Read the model definition and answer for the solid it produces. Units are mm, in the model's axes. Give positions to 0.01 mm unless a question says otherwise; leave off trailing zeros. Order: outer loops, then holes, each group sorted by start corner. A loop starts at its lowest first (then second) coordinate and runs counter-clockwise, first axis right, second up. Notation, with made-up numbers: (66.25, 74) -> (74.25, 74) arc R20 ccw to (74.25, 88) -> close; hole circle Ø2 at (42, -16). An arc over 180 degrees is marked (long way). Use one line per item in the form item = value.
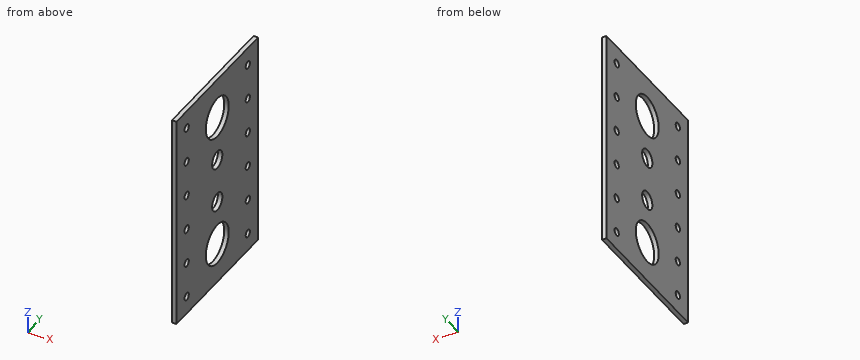
Autodesk Inventor part; units mm, degrees
ref_plane "YZ Plane" through (0, 0, 0) normal (1, 0, 0) x (0, 1, 0)
ref_plane "XZ Plane" through (0, 0, 0) normal (0, 1, 0) x (-1, 0, 0)
ref_plane "XY Plane" through (0, 0, 0) normal (0, 0, 1) x (1, 0, 0)
sketch "Sketch1" plane through (0, 0, 0) normal (1, 0, 0) x (0, 1, 0)
  line L0 (0, 0) -> (101.6, 0)
  line L1 (101.6, 0) -> (101.6, -152.4)
  line L2 (101.6, -152.4) -> (0, -152.4)
  line L3 (0, -152.4) -> (0, 0)
  circle A0 centre (50.8, -28.575) radius 14.2875
  circle A1 centre (50.8, -60.325) radius 6.35
  circle A2 centre (50.8, -92.075) radius 6.35
  circle A3 centre (50.8, -123.825) radius 14.2875
  line L4 (50.8, -28.575) -> (50.8, -123.825) construction
  circle A4 centre (88.9, -12.7) radius 2.65
  circle A5 centre (88.9, -38.1) radius 2.65
  circle A6 centre (88.9, -63.5) radius 2.65
  circle A7 centre (88.9, -88.9) radius 2.65
  circle A8 centre (88.9, -114.3) radius 2.65
  circle A9 centre (88.9, -139.7) radius 2.65
  circle A10 centre (12.7, -12.7) radius 2.65
  circle A11 centre (12.7, -38.1) radius 2.65
  circle A12 centre (12.7, -63.5) radius 2.65
  circle A13 centre (12.7, -88.9) radius 2.65
  circle A14 centre (12.7, -114.3) radius 2.65
  circle A15 centre (12.7, -139.7) radius 2.65
  point P0 (101.6, -76.2)
  point P1 (50.8, -76.2)
  point P2 (50.8, -152.4)
  dimension "d0" = 101.6
  dimension "d1" = 152.4
  dimension "d2" = 28.575
  dimension "d3" = 12.7
  dimension "d4" = 12.7
  dimension "d5" = 28.575
  dimension "d6" = 31.75
  dimension "d7" = 31.75
  dimension "d8" = 31.75
  dimension "d9" = 5.3
  dimension "d10" = 12.7
  dimension "d11" = 12.7
  dimension "d14" = 25.4
  dimension "d17" = 76.2
extrude "Extrusion1" add sketch "Sketch1" along normal blind 3.175
equation "\"d7\" = d6"
equation "\"d8\" = d7"
properties part number "CH-1-02-RearGearboxHousingMotorSide" material "Aluminum 6061"
Item 1: Straight lines are drawn through the part: L1, parallel to Y at x = 1.3, z = -139.7; L2, parallel to Z at x = 0.8, y = 50.8 (1 decimal); L3, parallel to Y at x = 2.05, z = -37. For each, find the intervals that lie inside material, in ascending order. Write a range as from..to.
Checks:
L1 = 0..10.05, 15.35..86.25, 91.55..101.6
L2 = -152.4..-138.1, -109.5..-98.4, -85.7..-66.7, -54..-42.9, -14.3..0
L3 = 0..10.29, 15.11..39.26, 62.34..86.49, 91.31..101.6
Item 2: The part is cut by section B-B on y = 50.8. Give the vertices of the cut face in (x, z) (1 decimal).
Checks:
outline = (0, -152.4) -> (3.2, -152.4) -> (3.2, -138.1) -> (0, -138.1) -> close; (0, -109.5) -> (3.2, -109.5) -> (3.2, -98.4) -> (0, -98.4) -> close; (0, -85.7) -> (3.2, -85.7) -> (3.2, -66.7) -> (0, -66.7) -> close; (0, -54) -> (3.2, -54) -> (3.2, -42.9) -> (0, -42.9) -> close; (0, -14.3) -> (3.2, -14.3) -> (3.2, 0) -> (0, 0) -> close
Item 3: Given pin 1 Ø23 at (y, z) = (50.8, -28.575) entering from +X; pin 2 Ø16.5 at (y, z) = (50.8, -60.325) entering from +X (3 decimals), each flat-ended and moving along its own axis, determine where each tip first touches the part or whether it passes through.
Checks:
pin_1 = through
pin_2 = 3.175
Item 4: The part is cut by section D-D on x = 1.95. State how many separate pieces and enclosed holes the cut face has, and give its area (3 significant figures).
Checks:
separate_pieces = 1
enclosed_holes = 16
area = 13,700 mm²
Item 5: The part is cut by section A-A on z = -12.7. Give the vertices of the cut face in (x, y) (3 decimals), and give its area (3 significant figures).
Checks:
outline = (0, 0) -> (3.175, 0) -> (3.175, 10.05) -> (0, 10.05) -> close; (0, 15.35) -> (3.175, 15.35) -> (3.175, 86.25) -> (0, 86.25) -> close; (0, 91.55) -> (3.175, 91.55) -> (3.175, 101.6) -> (0, 101.6) -> close
area = 289 mm²
Item 6: The part is cut by section C-C on z = -119.5. Give the vertices of the cut face in (x, y) (3 decimals).
Checks:
outline = (0, 0) -> (3.175, 0) -> (3.175, 37.183) -> (0, 37.183) -> close; (0, 64.417) -> (3.175, 64.417) -> (3.175, 101.6) -> (0, 101.6) -> close
